from build123d import *

# Parameters (mm, degrees)
ESQUISSE1_W             = 200
ESQUISSE1_H             = 28.284
BOSS_EXTRU_3_DEPTH      = 8
CHANFREIN1_SIZE         = 20
ESQUISSE4_R             = 2
ENL_V_MAT_EXTRU_1_DEPTH = 8
FILLET1_R               = 8
SKETCH2_R               = 1.5
SKETCH2_R_2             = 3.75
CUT_EXTRUDE1_DEPTH      = 8
FILLET9_R               = 1
FILLET10_R              = 1
FILLET4_R               = 4
FILLET5_R               = 4


# Some blends are built 0.0001 mm under size
with BuildPart() as part:
    # Esquisse1 → Boss.-Extru.3 (new body)
    with BuildSketch(Plane.XY):
        with Locations((100, 14.142)):
            Rectangle(ESQUISSE1_W, ESQUISSE1_H)
    extrude(amount=BOSS_EXTRU_3_DEPTH)

    # Chanfrein1
    # the kernel refuses this chamfer: 20 mm, written as the material it takes off along each edge
    with BuildSketch(Plane(origin=(200, -51.433659759, 8), x_dir=(0.027495876610586317, 0, -0.9996219169112968), z_dir=(0, 1, 0))) as chanfrein1_piece_1:
        Polygon((CHANFREIN1_SIZE * 0.999621916911, CHANFREIN1_SIZE * 0.0274958766106), (-CHANFREIN1_SIZE * 0.0274958766106, CHANFREIN1_SIZE * 0.999621916911), (0, 0), align=None)
    extrude(amount=131.151319519, mode=Mode.SUBTRACT)

    # Esquisse4 → Enlèv. mat.-Extru.1 (cut)
    with BuildSketch(Plane.XY.offset(8)):
        with Locations((178, 7.142)):
            Circle(ESQUISSE4_R)
        with Locations((178, 21.142)):
            Circle(ESQUISSE4_R)
    extrude(amount=-ENL_V_MAT_EXTRU_1_DEPTH, mode=Mode.SUBTRACT)

    # Fillet1
    fillet1_edges = [part.edges().sort_by_distance(p)[0] for p in [
        (0, 14.142, 0),
    ]]
    fillet(fillet1_edges, radius=FILLET1_R - 0.0001)  # a hair under: the kernel refuses the full size

    # Sketch2 → Cut-Extrude1 (cut)
    with BuildSketch(Plane.XY.offset(8)):
        with Locations((10.180485171, 7.281517741)):
            Circle(SKETCH2_R)
        with Locations((24.142857006, 20.883346587)):
            Circle(SKETCH2_R)
        with Locations((17.323003706, 13.918303783)):
            Circle(SKETCH2_R_2)
        Polygon((14.943517177, 18.243352736), (12.822196834, 16.122032392), (9.422196834, 19.522032392), (11.543517177, 21.643352736), align=None)
        Polygon((19.379761465, 9.564467761), (22.780003771, 6.164594852), (24.901208877, 8.286030428), (21.501081812, 11.685788108), align=None)
    extrude(amount=-CUT_EXTRUDE1_DEPTH, mode=Mode.SUBTRACT)

    # Fillet9
    fillet9_edges = [part.edges().sort_by_distance(p)[0] for p in [
        (9.422196834, 19.522032392, 4),
        (11.543517177, 21.643352736, 4),
        (14.943517177, 18.243352736, 4),
        (12.822196834, 16.122032392, 4),
    ]]
    fillet(fillet9_edges, radius=FILLET9_R)

    # Fillet10
    fillet10_edges = [part.edges().sort_by_distance(p)[0] for p in [
        (24.901208877, 8.286030428, 4),
        (22.780003771, 6.164594852, 4),
        (19.379761465, 9.564467761, 4),
        (21.501081812, 11.685788108, 4),
    ]]
    fillet(fillet10_edges, radius=FILLET10_R)

    # Fillet4
    fillet4_edges = [part.edges().sort_by_distance(p)[0] for p in [
        (97.99995, 0, 0),
        (2.343116461, 0, 2.343116461),
    ]]
    fillet(fillet4_edges, radius=FILLET4_R)

    # Fillet5
    fillet5_edges = [part.edges().sort_by_distance(p)[0] for p in [
        (97.99995, 28.284, 0),
        (2.343116461, 28.284, 2.343116461),
    ]]
    fillet(fillet5_edges, radius=FILLET5_R)


solid = part.part
Geometry check sheet. Reference: the model listing, model coordinates, mm. Round coordinates to 2 decimals unless told otherwise and drop trailing zeros. Write each loop counter-clockwise with the first axis right and the second up, starting at its lowest first coordinate (ties: lowest second). Pieces come first, ordered by that corner, then holes. Notation, with made-up numbers: (64.5, -15) -> (121.5, -15) arc R6 ccw to (121.5, -7) -> close; hole circle Ø2 at (88, -6.5). An arc over 180 degrees is marked (long way). One line per item, written item: value. Start each with the question number.
(1) Cross-section at A-A, the plane x = 178. Record the cut outline in (y, z), and give its area (3 significant figures).
(2) Draft check along X on faces 1 (the flat face through (184, 14, 4)), 2 (the cylindrical face through (19.05, 10.59, 4.06)), 3 (the cylindrical face through (99.26, 1.141, 1.203)). Enter one of: +X half, -X half, draft (parallel to the pull), parting line (faces both ways), or undercut.
(3) Cross-section at B-B, the plane z = 2.25. Give the number of separate pieces and of enclosed holes in the cut face, and give its area (3 significant figures).
(4) Go/stop test with flat-tipped pins: pin 1 Ø7 at (x, y) = (17.32, 13.92) entering from -Z; pin 2 Ø1.5 at (x, z) = (50, 1) entering from +Y. Record where each tip stops, or that it passes through.
(5) Scan lines: line 1 (X direction, y = 8, z = 7.75); line 2 (X direction, y = 6.75, z = 4); line 3 (Y direction, x = 178, z = 2). Record each from-to range of solid material in increasing order. Write a range as [from, to].
Answer:
1. outline: (0, 4) arc R4 ccw to (4, 0) -> (5.14, 0) -> (5.14, 8) -> (0, 8) -> close; (9.14, 0) -> (19.14, 0) -> (19.14, 8) -> (9.14, 8) -> close; (23.14, 0) -> (24.28, 0) arc R4 ccw to (28.28, 4) -> (28.28, 8) -> (23.14, 8) -> close
1. area: 155 mm²
2. face 1: +X half
2. face 2: undercut
2. face 3: draft
3. separate pieces: 1
3. enclosed holes: 7
3. area: 4,920 mm²
4. pin 1: through
4. pin 2: y = 27.59
5. line 1: [0, 8.86], [11.5, 20.94], [24.45, 176.19], [179.81, 180.25]
5. line 2: [1.07, 8.78], [11.58, 22.22], [23.34, 176.04], [179.96, 184]
5. line 3: [0.54, 5.14], [9.14, 19.14], [23.14, 27.75]
